from build123d import *

# Parameters (mm, degrees)
SKETCH1_W                 = 125
SKETCH1_H                 = 125
EXTRUDE1_DEPTH            = 43.18
SKETCH2_W                 = 99.6
SKETCH2_H                 = 99.6
CUT_EXTRUDE1_DEPTH        = 182.973933298
SKETCH3_W                 = 98.8148352
SKETCH3_H                 = 34.925
CUT_EXTRUDE2_DEPTH        = 182.973933298
SKETCH6_W                 = 98.8148352
SKETCH6_H                 = 34.925
CUT_EXTRUDE3_DEPTH        = 182.973933298
HOLE_WIZARD_2_D           = 6.6
HOLE_WIZARD_2_CBORE_D     = 11
HOLE_WIZARD_2_CBORE_DEPTH = 6.8


with BuildPart() as part:
    # Sketch1 → Extrude1 (new body)
    with BuildSketch(Plane(origin=(0, 0, 0), x_dir=(1, 0, 0), z_dir=(0, 1, 0))):
        with Locations((62.5, 62.5)):
            Rectangle(SKETCH1_W, SKETCH1_H)
    extrude(amount=EXTRUDE1_DEPTH)

    # Sketch2 → Cut-Extrude1 (cut, through all)
    with BuildSketch(Plane(origin=(0, 43.18, 0), x_dir=(-1, 0, 0), z_dir=(0, 1, 0))):
        with Locations((-62.5, -62.5)):
            Rectangle(SKETCH2_W, SKETCH2_H)
    extrude(amount=-CUT_EXTRUDE1_DEPTH, mode=Mode.SUBTRACT)

    # Sketch3 → Cut-Extrude2 (cut, through all)
    with BuildSketch(Plane.XY):
        with Locations((62.5, 17.4625)):
            Rectangle(SKETCH3_W, SKETCH3_H)
    extrude(amount=-CUT_EXTRUDE2_DEPTH, mode=Mode.SUBTRACT)

    # Sketch6 → Cut-Extrude3 (cut, through all)
    with BuildSketch(Plane(origin=(125, 0, 0), x_dir=(0, 0, -1), z_dir=(1, 0, 0))):
        with Locations((62.5, 17.4625)):
            Rectangle(SKETCH6_W, SKETCH6_H)
    extrude(amount=-CUT_EXTRUDE3_DEPTH, mode=Mode.SUBTRACT)

    # 打孔尺寸(%根据)内六角圆柱头螺钉的类型2 (through all)
    with Locations(Plane(origin=(0, 43.18, 0), x_dir=(-1, 0, 0), z_dir=(0, 1, 0))):
        with Locations((-6, -6), (-119, -6), (-119, -119), (-6, -119)):
            CounterBoreHole(HOLE_WIZARD_2_D / 2, HOLE_WIZARD_2_CBORE_D / 2, HOLE_WIZARD_2_CBORE_DEPTH)


solid = part.part
Part model, mm, in its own coordinate system. A direction names the side the tool comes from. Give positions to 0.01 mm unless a question says otherwise; leave off trailing zeros. Loops run counter-clockwise (first coordinate to the right, second up) from the corner with the lowest first, then second, coordinate; pieces in that order, holes last. Notation, with made-up numbers: M 1.25,9 L 24.25,9 A18 ccw 24.25,35 Z; hole C 44.25,77.25 d4. An arc over 180 degrees is marked long. Put each result on its own line as item: value. Start each with the question number.
1) Saw through at B-B (x = 119). List the corners of the cut face in (y, z) (3 decimals).
2) Saw through at A-A (y = 31). List the corners of the cut face in (x, z), then the cut area to 3 significant figures.
3) Probe probe 1 along Z at (x, y) = (119, 18); probe 2 along Z at (x, y) = (6, 38.5); probe 3 along Z at (x, y) = (50, 35). List the from-to ranges inside material, lowest first.
4) Saw through at C-C (z = -6). List the corners of the cut face in (x, y) (3 decimals), then the cut area to 3 significant figures.
5) Pull direction Z, two halves, no side cores. Call faces 1 (the flat face through (9.4, 0, -6.6)), 2 (the flat face through (62, 36, 0)), 3 (the cylindrical face through (5.28, 17.94, -122.22)): +Z half, -Z half, draft (parallel to the pull), parting line (faces both ways), or undercut.
6) Flat gauge pins, fed straight in: pin 1 (14 mm diameter, centred on x = 119, z = -60.5, fed in from -Y) (3 decimals); pin 2 (9 mm diameter, centred on x = 119, z = -6, fed in from +Y); pin 3 (1 mm diameter, centred on x = 110, z = -68.5, fed in from +Y). Where does each tip first touch, or does it go through?
7) 3-axis set-ups, long thin cutter, end or side, ignore diameter. For faces 4 (the flat face through (112.3, 39, -63)), 5 (the flat face through (13.093, 17, -6)), 6 (the flat face through (2, 36.38, -6)), 7 (the flat face through (119, 17, -13.093)): which of +Z, -Z, +X, -X, +Y, -Y reach the whole face in a straight line?
8) Saw through at D-D (x = 97). List the corners of the cut face in (y, z) (3 decimals), then the cut area to 3 significant figures.
Numbers:
1. outline: M 0,-125 L 43.18,-125 L 43.18,-124.5 L 36.38,-124.5 L 36.38,-122.3 L 0,-122.3 Z; M 0,-115.7 L 36.38,-115.7 L 36.38,-113.5 L 43.18,-113.5 L 43.18,-11.5 L 36.38,-11.5 L 36.38,-9.3 L 0,-9.3 L 0,-13.093 L 34.925,-13.093 L 34.925,-111.907 L 0,-111.907 Z; M 0,-2.7 L 36.38,-2.7 L 36.38,-0.5 L 43.18,-0.5 L 43.18,0 L 0,0 Z
2. outline: M 0,-125 L 13.09,-125 L 13.09,-112.3 L 12.7,-112.3 L 12.7,-111.91 L 0,-111.91 Z; M 0,-13.09 L 12.7,-13.09 L 12.7,-12.7 L 13.09,-12.7 L 13.09,0 L 0,0 Z; M 111.91,-125 L 125,-125 L 125,-111.91 L 112.3,-111.91 L 112.3,-112.3 L 111.91,-112.3 Z; M 111.91,-12.7 L 112.3,-12.7 L 112.3,-13.09 L 125,-13.09 L 125,0 L 111.91,0 Z; hole C 6,-119 d6.6; hole C 6,-6 d6.6; hole C 119,-119 d6.6; hole C 119,-6 d6.6
2. area: 548 mm^2
3. probe 1: -125 to -122.3, -115.7 to -111.91, -13.09 to -9.3, -2.7 to 0
3. probe 2: -125 to -124.5, -113.5 to -11.5, -0.5 to 0
3. probe 3: -125 to -112.3, -12.7 to 0
4. outline: M 0,0 L 2.7,0 L 2.7,36.38 L 0.5,36.38 L 0.5,43.18 L 0,43.18 Z; M 9.3,0 L 13.093,0 L 13.093,34.925 L 111.907,34.925 L 111.907,0 L 115.7,0 L 115.7,36.38 L 113.5,36.38 L 113.5,43.18 L 11.5,43.18 L 11.5,36.38 L 9.3,36.38 Z; M 122.3,0 L 125,0 L 125,43.18 L 124.5,43.18 L 124.5,36.38 L 122.3,36.38 Z
4. area: 1,320 mm^2
5. face 1: draft
5. face 2: +Z half
5. face 3: undercut
6. pin 1: y = 34.925
6. pin 2: y = 36.38
6. pin 3: through
7. face 4: +Y, -Y
7. face 5: +Z, -Z, -Y
7. face 6: +Y
7. face 7: +X, -X, -Y
8. outline: M 34.925,-125 L 43.18,-125 L 43.18,-112.3 L 34.925,-112.3 Z; M 34.925,-12.7 L 43.18,-12.7 L 43.18,0 L 34.925,0 Z
8. area: 210 mm^2
